from build123d import *

# Parameters (mm, degrees)
SKETCH1_W           = 7
SKETCH1_H           = 7
BOSS_EXTRUDE1_DEPTH = 3
SKETCH3_W           = 10
SKETCH3_H           = 10
BOSS_EXTRUDE2_DEPTH = 12
BOSS_EXTRUDE4_DEPTH = 4
SKETCH7_W           = 10
SKETCH7_H           = 10
BOSS_EXTRUDE6_DEPTH = 4
SKETCH8_W           = 10
SKETCH8_H           = 4
BOSS_EXTRUDE7_DEPTH = 53.5


with BuildPart() as part:
    # Sketch1 → Boss-Extrude1 (new body)
    with BuildSketch(Plane(origin=(0, 0, 0), x_dir=(1, 0, 0), z_dir=(0, 1, 0))):
        Rectangle(SKETCH1_W, SKETCH1_H)
    extrude(amount=BOSS_EXTRUDE1_DEPTH)

    # Sketch3 → Boss-Extrude2 (add)
    with BuildSketch(Plane(origin=(0, 3, 0), x_dir=(1, 0, 0), z_dir=(0, 1, 0))):
        Rectangle(SKETCH3_W, SKETCH3_H)
    extrude(amount=BOSS_EXTRUDE2_DEPTH)

    # Sketch7 → Boss-Extrude6 (add)
    with BuildSketch(Plane(origin=(0, 15, 0), x_dir=(1, 0, 0), z_dir=(0, 1, 0))):
        Rectangle(SKETCH7_W, SKETCH7_H)
    extrude(amount=BOSS_EXTRUDE6_DEPTH)



with BuildPart() as body_2:
    # Sketch4 → Boss-Extrude4 (new body)
    with BuildSketch(Plane(origin=(0, 15, 0), x_dir=(1, 0, 0), z_dir=(0, 1, 0))):
        Polygon((105, 43.294473551), (105, 55.294473551), (95, 55.294473551), (95, 43.294473551), (58.5, 43.294473551), (58.5, -43.294473551), (95, -43.294473551), (95, -55.294473551), (105, -55.294473551), (105, -43.294473551), (141.5, -43.294473551), (141.5, -5), (153.5, -5), (153.5, 5), (141.5, 5), (141.5, 43.294473551), align=None)
    extrude(amount=BOSS_EXTRUDE4_DEPTH)


with BuildPart() as part_1:
    add(part.part)

    add(body_2.part)  # Boss-Extrude7 merges body 2
    # Sketch8 → Boss-Extrude7 (add)
    with BuildSketch(Plane(origin=(5, 0, 0), x_dir=(0, 0, -1), z_dir=(1, 0, 0))):
        with Locations((0, 17)):
            Rectangle(SKETCH8_W, SKETCH8_H)
    extrude(amount=BOSS_EXTRUDE7_DEPTH)


solid = part_1.part
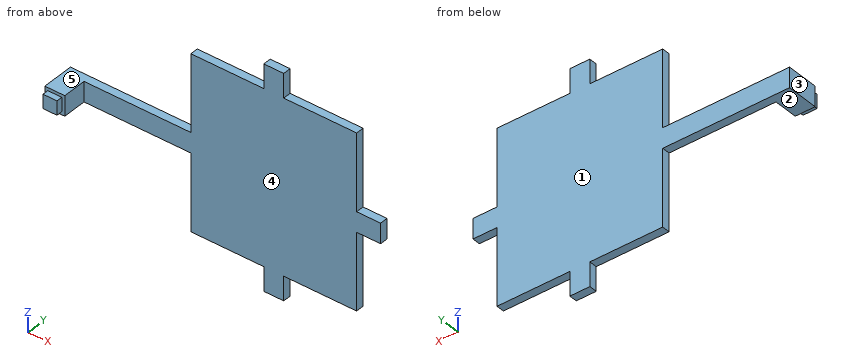
For this review, take the finished solid that the model builds, in its own axes (mm). Face numbers are marked on the shaded views. A direction names the side the tool comes from. Round coordinates to 2 decimals unless told otherwise and drop trailing zeros. Write each loop counter-clockwise with the first axis right and the second up, starting at its lowest first coordinate (ties: lowest second). Pieces come first, ordered by that corner, then holes. Notation, with made-up numbers: M -15,19 L 11,19 A21 ccw 11,24 Z; hole C -9.75,-7 d4. An arc over 180 degrees is marked long. Write item = value, one per line. Start each with the question number.
(1) For the marked faces 1, 2, 3, 4 and 5, list the 3-axis set-ups (+Z, -Z, +X, -X, +Y, -Y) from which the entire face can be reached by the end or side of a thin tool; tool diameter is ignored.
(2) We need section B-B (y = 12.25). Give the boundary of the cut face in (x, z).
(3) For line 1 along X through (y, z) = (15.75, 13.5); line 2 along X through (y, z) = (9.5, 3); line 3 along Y through (x, z) = (81.5, -14), list the stretches that pass through material, from the lowest coordinate up.
(4) We need section A-A (z = 1). Give the boundary of the cut face in (x, y), then the cut area to 3 significant figures.
(5) Clearance check with flat-ended pins moving along their axes: pin 1 Ø2.5 at (x, y) = (1.5, 1) entering from -Z; pin 2 Ø2 at (y, z) = (18, -26.5) entering from +X; pin 3 Ø1.2 at (x, y) = (123.5, 17) entering from -Z. State where each tip first meets the part, or that it passes through.
(6) We need section C-C (x = 16). Give the boundary of the cut face in (y, z).
Results found:
q1.face_1 = +Z, -Z, +X, -X, +Y
q1.face_2 = -Z, -X, +Y, -Y
q1.face_3 = +Z, -Z, -X, +Y, -Y
q1.face_4 = +Z, -Z, +X, -Y
q1.face_5 = +Z, -X, +Y, -Y
q2.outline = M -5,-5 L 5,-5 L 5,5 L -5,5 Z
q3.line_1 = 58.5 to 141.5
q3.line_2 = -5 to 5
q3.line_3 = 15 to 19
q4.outline = M -5,3 L -3.5,3 L -3.5,0 L 3.5,0 L 3.5,3 L 5,3 L 5,15 L 153.5,15 L 153.5,19 L -5,19 Z
q4.area = 775 mm²
q5.pin_1 = -3.5
q5.pin_2 = 141.5
q5.pin_3 = -43.29
q6.outline = M 15,-5 L 19,-5 L 19,5 L 15,5 Z
